Verification items for the finished model (mm, model axes). Face numbers are marked on the shaded views. A direction names the side the tool comes from. Round coordinates to 2 decimals unless told otherwise and drop trailing zeros. Write each loop counter-clockwise with the first axis right and the second up, starting at its lowest first coordinate (ties: lowest second). Pieces come first, ordered by that corner, then holes.
Autodesk Inventor part; units mm, degrees
ref_plane "YZ Plane" through (0, 0, 0) normal (1, 0, 0) x (0, 1, 0)
ref_plane "XZ Plane" through (0, 0, 0) normal (0, 1, 0) x (-1, 0, 0)
ref_plane "XY Plane" through (0, 0, 0) normal (0, 0, 1) x (1, 0, 0)
sketch "Sketch1" plane through (0, 0, 0) normal (0, 0, 1) x (1, 0, 0)
  line L0 (0, 0) -> (70, 0)
  line L1 (70, 0) -> (70, 55)
  line L2 (70, 55) -> (0, 55)
  line L3 (0, 55) -> (0, 0)
  dimension "d0" = 70
  dimension "d1" = 55
extrude "Extrusion1" add sketch "Sketch1" along normal blind 8
sketch "Sketch2" plane through (0, 0, 8) normal (0, 0, 1) x (1, 0, 0)
  circle A0 centre (11, 5) radius 1.75
  circle A1 centre (65, 5) radius 1.75
  circle A2 centre (11, 46) radius 1.75
  circle A3 centre (65, 46) radius 1.75
  line L0 (0, 55) -> (0, 0)
  line L1 (0, 0) -> (70, 0)
  line L2 (70, 55) -> (0, 55)
  line L3 (70, 0) -> (70, 55)
  dimension "d4" = 3.5
  dimension "d5" = 3.5
  dimension "d6" = 3.5
  dimension "d7" = 3.5
  dimension "d8" = 11
  dimension "d9" = 5
  dimension "d10" = 9
  dimension "d11" = 5
extrude "Extrusion2" cut sketch "Sketch2" against normal blind 40 contours A0 | A1 | A2 | A3
sketch "Sketch3" plane through (0, 0, 0) normal (0, 0, -1) x (-1, 0, 0)
  circle A0 centre (-22, 33) radius 11.5
  line L0 (0, 55) -> (0, 0)
  line L1 (-70, 55) -> (0, 55)
  dimension "d14" = 23
  dimension "d15" = 22
  dimension "d16" = 22
extrude "Extrusion3" cut sketch "Sketch3" against normal blind 35
sketch "Sketch4" plane through (0, 0, 0) normal (0, 0, -1) x (-1, 0, 0)
  circle A0 centre (-22, 33) radius 11.5
  point P0 (0, 0)
  point P1 (-6.5, 48.5)
  point P2 (-37.5, 48.5)
  point P3 (-37.5, 17.5)
  point P4 (-6.5, 17.5)
  dimension "d19" = 15.5
  dimension "d20" = 15.5
  dimension "d21" = 15.5
  dimension "d22" = 15.5
hole "Hole1" at (6.5, 17.5, 0) at (37.5, 17.5, 0) at (37.5, 48.5, 0) direction (0, 0, 1) diameter 3.5 end through all
sketch "Sketch5" plane through (0, 0, 0) normal (0, 0, -1) x (-1, 0, 0)
  arc A0 (-46, 45.5) -> (-46, 5.5) centre (-46, 25.5) ccw
  line L0 (-46, 45.5) -> (-44, 45.5)
  line L1 (-44, 45.5) -> (-44, 5.5)
  line L2 (-44, 5.5) -> (-46, 5.5)
  line L3 (-70, 0) -> (-70, 55)
  point P0 (0, 0)
  dimension "d30" = 40
  dimension "d32" = 25.5
  dimension "d33" = 24
  dimension "d34" = 26
extrude "Extrusion4" cut sketch "Sketch5" against normal blind 35
sketch "Sketch6" plane through (0, 0, 8) normal (0, 0, 1) x (1, 0, 0)
  arc A0 (46, 5.5) -> (46, 45.5) centre (46, 25.5) ccw
  line L0 (46, 5.5) -> (44, 5.5)
  line L1 (44, 5.5) -> (44, 45.5)
  line L2 (44, 45.5) -> (46, 45.5)
  arc A1 (46, 4.5) -> (46, 46.5) centre (46, 25.5) ccw
  line L3 (46, 4.5) -> (43, 4.5)
  line L4 (43, 4.5) -> (43, 46.5)
  line L5 (43, 46.5) -> (46, 46.5)
  line L6 (70, 0) -> (70, 55)
  point P0 (0, 0)
  dimension "d37" = 42
  dimension "d38" = 27
extrude "Extrusion5" add sketch "Sketch6" along normal blind 37.5
equation "\"d5\" = d4"
equation "\"d6\" = d4"
equation "\"d7\" = d4"
properties part number "BLOQUE_PARA_MOTOR"
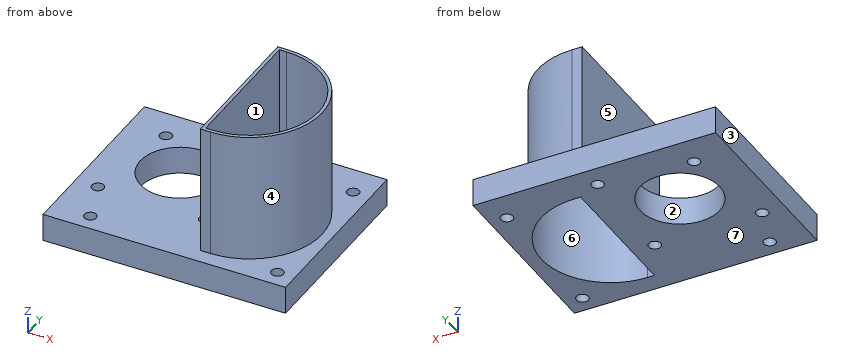
Q1. Sectioned sample at C-C (y = 25.5). Enter the section's corners in (x, z), plus the area to 3 significant figures.
Recorded:
outline: (0, 0) - (13.28, 0) - (13.28, 8) - (0, 8) - close; (30.72, 0) - (44, 0) - (44, 45.5) - (43, 45.5) - (43, 8) - (30.72, 8) - close; (66, 0) - (70, 0) - (70, 8) - (67, 8) - (67, 45.5) - (66, 45.5) - close
area: 320 mm2
Q2. Sectioned sample at D-D (x = 51.5). Enter the section's corners in (y, z).
Recorded:
outline: (0, 0) - (6.27, 0) - (6.27, 45.5) - (5.23, 45.5) - (5.23, 8) - (0, 8) - close; (44.73, 0) - (55, 0) - (55, 8) - (45.77, 8) - (45.77, 45.5) - (44.73, 45.5) - close
Q3. Release check for a two-part mould opening along Y. For the marked faces 1, 2, 3 and 4 record: released by +Y, released by -Y, zero draft, split by the parting line, or undercut.
Recorded:
face 1: undercut
face 2: undercut
face 3: zero draft
face 4: split by the parting line
Q4. Sectioned sample at B-B (x = 6.5). Enter the section's corners in (y, z).
Recorded:
outline: (0, 0) - (15.75, 0) - (15.75, 8) - (0, 8) - close; (19.25, 0) - (55, 0) - (55, 8) - (19.25, 8) - close
Q5. Sectioned sample at A-A (z = 42). Enter the section's corners in (x, y), plus the area to 3 significant figures.
Recorded:
outline: (43, 4.5) - (46, 4.5) arc R21 ccw to (46, 46.5) - (43, 46.5) - close; hole (44, 5.5) - (46, 5.5) arc R20 ccw to (46, 45.5) - (44, 45.5) - close
area: 110 mm2
Q6. Material ranges on line 1 along Y through (x, z) = (6.5, 6); line 2 along X through (y, z) = (17.5, 4); line 3 along Y through (x, z) = (22, 5), recorded low to high.
Recorded:
line 1: y = 0 to 15.75, 19.25 to 55
line 2: x = 0 to 4.75, 8.25 to 35.75, 39.25 to 44, 64.33 to 70
line 3: y = 0 to 21.5, 44.5 to 55
Q7. Depth check by flat-ended pin: P1, Ø4, axis at y = 43.5, z = 39, coming from the -X side; P2, Ø4.5, axis at x = 11, y = 46, coming from the +Z side; P3, Ø0.9, axis at x = 45, z = 33, coming from the +Y side; P4, Ø4.5, axis at x = 6.5, y = 17.5, coming from the -Z side. Enter the tip coordinate at first touch or a pass-through.
Recorded:
P1: stops at x = 43
P2: stops at z = 8
P3: stops at y = 46.5
P4: stops at z = 0
Q8. Tool access check on the marked faces 5, 6 and 7. Record the directions out of +Z, -Z, +X, -X, +Y, -Y that give a thin tool (end or side, any length) a straight path to the whole face; none if there is none.
Recorded:
face 5: +Z, -X, +Y, -Y
face 6: +Z, -Z
face 7: -Z, +X, -X, +Y, -Y
